```python
from build123d import *

# Parameters (mm, degrees)
ESQUISSE1_W                  = 40
ESQUISSE1_H                  = 75
BOSS_EXTRU_1_DEPTH           = 4
ENL_V_MAT_EXTRU_1_DEPTH      = 5
ESQUISSE3_R                  = 6.5
ESQUISSE3_R_2                = 3
ENL_V_MAT_EXTRU_2_DEPTH      = 5
CONG_1_R                     = 5
ESQUISSE4_R                  = 3.5
ENL_V_MAT_EXTRU_3_DEPTH      = 5
ENL_V_MAT_EXTRU_4_DEPTH      = 1
ENL_V_MAT_EXTRU_4_DEPTH_BACK = 5
ESQUISSE6_W                  = 3.826832881
ESQUISSE6_H                  = 13.310723064
ESQUISSE6_H_2                = 14.142643256
BOSS_EXTRU_2_DEPTH           = 4
CONG_2_R                     = 3


with BuildPart() as part:
    # Esquisse1 → Boss.-Extru.1 (new body)
    with BuildSketch(Plane.XY):
        with Locations((20, 37.5)):
            Rectangle(ESQUISSE1_W, ESQUISSE1_H)
    extrude(amount=BOSS_EXTRU_1_DEPTH)

    # Esquisse2 → Enlèv. mat.-Extru.1 (cut, through all)
    with BuildSketch(Plane.XY.offset(4)):
        Polygon((0, 16.5), (0, 49.5), (14, 44), (14, 22), align=None)
    extrude(amount=-ENL_V_MAT_EXTRU_1_DEPTH, mode=Mode.SUBTRACT)

    # Esquisse3 → Enlèv. mat.-Extru.2 (cut, through all)
    with BuildSketch(Plane.XY.offset(4)):
        with Locations((9, 66)):
            Circle(ESQUISSE3_R)
        with Locations((9, 9)):
            Circle(ESQUISSE3_R)
        with Locations((11, 51.890523543)):
            Circle(ESQUISSE3_R_2)
    extrude(amount=-ENL_V_MAT_EXTRU_2_DEPTH, mode=Mode.SUBTRACT)

    # Congé1
    cong_1_edges = [part.edges().sort_by_distance(p)[0] for p in [
        (0, 16.5, 2),
        (0, 49.5, 2),
        (14, 44, 2),
        (14, 22, 2),
        (0, 75, 2),
        (40, 75, 2),
        (40, 0, 2),
        (0, 0, 2),
    ]]
    fillet(cong_1_edges, radius=CONG_1_R)

    # Esquisse4 → Enlèv. mat.-Extru.3 (cut, through all)
    with BuildSketch(Plane.XY.offset(4)):
        with Locations((33, 69)):
            Circle(ESQUISSE4_R)
        with Locations((33, 6)):
            Circle(ESQUISSE4_R)
    extrude(amount=-ENL_V_MAT_EXTRU_3_DEPTH, mode=Mode.SUBTRACT)

    # Esquisse5 → Enlèv. mat.-Extru.4 (cut, two sides)
    with BuildSketch(Plane.XY.offset(4)) as enl_v_mat_extru_4_sk:
        with BuildLine():
            Line((28, 58), (28, 17.901446768))
            ThreePointArc((28, 17.901446768), (33, 11.919389183), (38, 17.901446768))
            Line((38, 17.901446768), (38, 58))
            ThreePointArc((38, 58), (33, 63), (28, 58))
        make_face()
    extrude(amount=ENL_V_MAT_EXTRU_4_DEPTH, mode=Mode.SUBTRACT)
    extrude(enl_v_mat_extru_4_sk.sketch, amount=-ENL_V_MAT_EXTRU_4_DEPTH_BACK, mode=Mode.SUBTRACT)

    # Esquisse6 → Boss.-Extru.2 (add)
    with BuildSketch(Plane.XY.offset(4)):
        with Locations((16.413416441, 65.03655834)):
            Rectangle(ESQUISSE6_W, ESQUISSE6_H)
        with Locations((16.413416441, 9.381097526)):
            Rectangle(ESQUISSE6_W, ESQUISSE6_H_2)
    extrude(amount=-BOSS_EXTRU_2_DEPTH)

    # Congé2
    cong_2_edges = [part.edges().sort_by_distance(p)[0] for p in [
        (14.5, 69.464101615, 2),
        (14.5, 62.535898385, 2),
        (14.5, 12.464101615, 2),
        (14.5, 5.535898385, 2),
    ]]
    fillet(cong_2_edges, radius=CONG_2_R)


solid = part.part
```
The model under review builds one solid part; all positions refer to its coordinate system, in mm. A direction names the side the tool comes from. Round coordinates to 2 decimals unless told otherwise and drop trailing zeros. Loops run counter-clockwise (first coordinate to the right, second up) from the corner with the lowest first, then second, coordinate; pieces in that order, holes last. Notation, with made-up numbers: (-29, 39.25) - (5, 39.25) arc R22 cw to (5, 62.25) - close; hole circle Ø10 at (3.25, 19). An arc over 180 degrees is marked (long way). Use a Markdown table: item, result. Add a question column.
Q1. Machinability: for faces 4 (the face through (20, 0, 2)), 5 (the face through (13.155, 43.373, 1.972)), 6 (the face through (14.284, 62.432, 2.028)), which of the approach directions +Z, -Z, +X, -X, +Y, -Y give a long, thin tool a straight path to every point of the face, cutting with its end or side? Answer none if there is none.
Q2. Insertion check: pin 1 Ø6 at (x, y) = (33, 17) entering from -Z. The pin has a flat end and moves straight along its axis. Give the tip position at first contact, or say it passes through.
Q3. Add section C-C (y = 60.5). State the section outline as (x, z) points, plus the area to 3 significant figures.
Q4. Add section A-A (y = 17). State the section outline as (x, z) points, plus the area to 3 significant figures.
Q5. Add section D-D (z = 1.4). State how many separate pieces and enclosed holes the cut face has, plus the area to 3 significant figures.
Q6. Add section B-B (x = 9). State the section outline as (y, z) points, plus the area to 3 significant figures.
Q7. For probe 1 along Y at (x, z) = (33, 3); probe 2 along X at (y, z) = (37, 3.5); probe 3 along Y at (x, z) = (9, 2.1), list the stretches that pass through material, from the lowest coordinate up.
Q8. The part is to be moulded in two halves that separate along X. For faces 1 (the face through (20, 38, 0)), 2 (the face through (13.11, 22.56, 1.97)), 3 (the face through (14.5, 66, 2)), say which applies: pulls with the +X half, pulls with the -X half, needs draft (parallel to the pull), parting line crosses it, or undercut.
Worked answers:
| question | item | result |
|---|---|---|
| 1 | face 4 | +Z, -Z, +X, -X, -Y |
| 1 | face 5 | +Z, -Z, -X |
| 1 | face 6 | +Z, -Z |
| 2 | pin 1 | through |
| 3 | outline | (0, 0) - (5.54, 0) - (5.54, 4) - (0, 4) - close; (12.46, 0) - (28.67, 0) - (28.67, 4) - (12.46, 4) - close; (37.33, 0) - (40, 0) - (40, 4) - (37.33, 4) - close |
| 3 | area | 97.6 mm² |
| 4 | outline | (1.88, 0) - (27.92, 0) - (27.92, 4) - (1.88, 4) - close; (38.08, 0) - (40, 0) - (40, 4) - (38.08, 4) - close |
| 4 | area | 112 mm² |
| 5 | separate pieces | 1 |
| 5 | enclosed holes | 6 |
| 5 | area | 1,740 mm² |
| 6 | outline | (0, 0) - (2.5, 0) - (2.5, 4) - (0, 4) - close; (15.5, 0) - (20.04, 0) - (20.04, 4) - (15.5, 4) - close; (45.96, 0) - (49.65, 0) - (49.65, 4) - (45.96, 4) - close; (54.13, 0) - (59.5, 0) - (59.5, 4) - (54.13, 4) - close; (72.5, 0) - (75, 0) - (75, 4) - (72.5, 4) - close |
| 6 | area | 74.4 mm² |
| 7 | probe 1 | 0 to 2.5, 9.5 to 11.92, 63 to 65.5, 72.5 to 75 |
| 7 | probe 2 | 14 to 28, 38 to 40 |
| 7 | probe 3 | 0 to 2.5, 15.5 to 20.04, 45.96 to 49.65, 54.13 to 59.5, 72.5 to 75 |
| 8 | face 1 | needs draft |
| 8 | face 2 | pulls with the -X half |
| 8 | face 3 | undercut |
